Can you work these out from the model? Positions are in its coordinate system, mm. A direction names the side the tool comes from. Coordinates: 2 decimals unless noted, no trailing zeros. Order: outer loops, then holes, each group sorted by start corner. A loop starts at its lowest first (then second) coordinate and runs counter-clockwise, first axis right, second up. Notation, with made-up numbers: (69, 27.25) -> (83, 27.25) arc R10 cw to (83, 39.25) -> close; hole circle Ø1 at (47.25, 34.25). An arc over 180 degrees is marked (long way). Use a Markdown table: item, result. Add a question column.
1. If I drill on line 1 along Y through (x, z) = (36.5, 6); line 2 along Y through (x, z) = (6, 10.25); line 3 along X through (y, z) = (-7.5, 13.25), over which ranges is the centre line in solid material (lowest first)? Write a range as from..to.
2. Suppose I cut it at A-A, the plane z = 10.75. List the corners of the cut face in (x, y) for me.
3. For faces 4 (the cylindrical face through (-74.14, -10.26, 14.1)), 5 (the flat face through (-1.05, -21.617, 8.967)), which set-ups out of +Z, -Z, +X, -X, +Y, -Y let a thin tool reach every point of the face, with its end or its side?
4. We'd pull the mould along Z, two halves only. Please class faces 1 (the flat face through (-1, 0, 6)), 2 (the flat face through (-1, -11, 15)), 3 (the flat face through (-1.05, -24.47, 3.08)): pulls with the +Z half, pulls with the -Z half, needs draft (parallel to the pull), parting line crosses it, or undercut.
5. Suppose I cut it at B-B, the plane x = 42.5. List the corners of the cut face in (y, z) for me, then the cut area to 3 significant figures.
6. For pin 1 Ø6 at (y, z) = (-23, 6) entering from +X, with a flat end and sliding along its axis, tell me the tip position at first contact or that it passes through.
```python
from build123d import *

# Parameters (mm, degrees)
F0_W     = 150
F0_H     = 40
F1_DEPTH = 15
F3_DEPTH = 150
F4_R     = 3


with BuildPart() as f1:
    # F0 (on Top) → F1 (new body)
    with BuildSketch(Plane.XY):
        with Locations((0, -20)):
            Rectangle(F0_W, F0_H)
    extrude(amount=F1_DEPTH)

    # F2 (on face) → F3 (cut)
    with BuildSketch(Plane(origin=(-75, 0, 0), x_dir=(0, -1, 0), z_dir=(-1, 0, 0))):
        Polygon((22.588190451, 15), (20, 15), (23.2792044265, 2.7618424718), (25.6940189923, 3.4088900845), align=None)
    extrude(amount=-F3_DEPTH, mode=Mode.SUBTRACT)

    # F4
    f4_edges = [f1.edges().sort_by_distance(p)[0] for p in [
        (0, 0, 15),
        (-75, -10, 15),
        (75, -10, 15),
        (75, -31.294095, 15),
        (0, -40, 15),
        (-75, -31.294095, 15),
    ]]
    fillet(f4_edges, radius=F4_R)


solid = f1.part
```
Worked out:
| question | item | result |
|---|---|---|
| 1 | line 1 | y = -40..-25, -22.41..0 |
| 1 | line 2 | y = -40..-23.86, -21.27..0 |
| 1 | line 3 | x = -74.73..74.73 |
| 2 | outline | (-75, -40) -> (75, -40) -> (75, -23.73) -> (-75, -23.73) -> close; (-75, -21.14) -> (75, -21.14) -> (75, 0) -> (-75, 0) -> close |
| 3 | face 4 | +Z, -X, +Y, -Y |
| 3 | face 5 | +X, -X |
| 4 | face 1 | needs draft |
| 4 | face 2 | pulls with the +Z half |
| 4 | face 3 | undercut |
| 5 | outline | (-40, 0) -> (0, 0) -> (0, 12) arc R3 ccw to (-3, 15) -> (-20, 15) -> (-23.28, 2.76) -> (-25.69, 3.41) -> (-22.59, 15) -> (-37, 15) arc R3 ccw to (-40, 12) -> close |
| 5 | area | 565 mm² |
| 6 | pin 1 | stops at x = 75 |
